Work out the finished part from the listing and answer in its coordinate system (mm). A direction names the side the tool comes from. Round coordinates to 2 decimals unless told otherwise and drop trailing zeros. Write each loop counter-clockwise with the first axis right and the second up, starting at its lowest first coordinate (ties: lowest second). Pieces come first, ordered by that corner, then holes. Notation, with made-up numbers: (-36, 31.5) - (-10, 31.5) arc R6 ccw to (-10, 36.5) - close; hole circle Ø11 at (25.5, 48.5). An arc over 180 degrees is marked (long way). Answer as a JSON object with one key per item and string values.
```python
from build123d import *

# Parameters (mm, degrees)
ESBO_O1_W                  = 69
ESBO_O1_H                  = 31.5
RESSALTO_EXTRUS_O1_DEPTH   = 6
ESBO_O2_W                  = 5
ESBO_O2_H                  = 19
RESSALTO_EXTRUS_O2_DEPTH   = 20
ESBO_O3_W                  = 5
ESBO_O3_H                  = 7
CORTE_EXTRUS_O1_DEPTH      = 10
ESBO_O4_W                  = 4
ESBO_O4_H                  = 31.5
RESSALTO_EXTRUS_O3_DEPTH   = 20
CORTE_EXTRUS_O2_DEPTH      = 4
ESBO_O6_W                  = 4
ESBO_O6_H                  = 6
RESSALTO_EXTRUS_O4_DEPTH   = 50
ESBO_O7_W                  = 4
ESBO_O7_H                  = 63
RESSALTO_EXTRUS_O5_DEPTH   = 10
CORTE_EXTRUS_O3_DEPTH      = 144.957450913
CORTE_EXTRUS_O3_DEPTH_BACK = 144.957450913
ESBO_O8_R                  = 3
ESBO_O13_W                 = 100
ESBO_O13_H                 = 4
RESSALTO_EXTRUS_O6_DEPTH   = 53


with BuildPart() as part:
    # Esboço1 → Ressalto-extrusão1 (new body)
    with BuildSketch(Plane.XY):
        with Locations((-34.5, -15.931977108)):
            Rectangle(ESBO_O1_W, ESBO_O1_H)
    extrude(amount=RESSALTO_EXTRUS_O1_DEPTH)

    # Esboço2 → Ressalto-extrusão2 (add)
    with BuildSketch(Plane.XY.offset(6)):
        with Locations((-60, -22.181977108)):
            Rectangle(ESBO_O2_W, ESBO_O2_H)
    extrude(amount=RESSALTO_EXTRUS_O2_DEPTH)

    # Esboço3 → Corte-extrusão1 (cut)
    with BuildSketch(Plane.XY.offset(26)):
        with Locations((-60, -22.181977108)):
            Rectangle(ESBO_O3_W, ESBO_O3_H)
    extrude(amount=-CORTE_EXTRUS_O1_DEPTH, mode=Mode.SUBTRACT)

    # Esboço4 → Ressalto-extrusão3 (add)
    with BuildSketch(Plane.XY.offset(6)):
        with Locations((-52, -15.931977108)):
            Rectangle(ESBO_O4_W, ESBO_O4_H)
    extrude(amount=RESSALTO_EXTRUS_O3_DEPTH)

    # Esboço5 → Corte-extrusão2 (cut)
    with BuildSketch(Plane(origin=(-50, 0, 0), x_dir=(0, 0, -1), z_dir=(1, 0, 0))):
        Polygon((-22, -25.681977108), (-6, -25.681977108), (-6, -0.181977108), (-22, -0.181977108), (-22, -6.181977108), align=None)
    extrude(amount=-CORTE_EXTRUS_O2_DEPTH, mode=Mode.SUBTRACT)

    # Esboço6 → Ressalto-extrusão4 (add)
    with BuildSketch(Plane(origin=(-50, 0, 0), x_dir=(0, 0, -1), z_dir=(1, 0, 0))):
        with Locations((-24, -28.681977108)):
            Rectangle(ESBO_O6_W, ESBO_O6_H)
    extrude(amount=RESSALTO_EXTRUS_O4_DEPTH)

    # Espelhar10: part across plane


with BuildPart() as part_1:
    add(part.part)
    add(part.part.mirror(Plane.ZX.offset(-0.181977108)))

    # Espelhar11: part across plane


with BuildPart() as part_2:
    add(part_1.part)
    add(part_1.part.mirror(Plane(origin=(0, 0, 0), x_dir=(0, 0, 1), z_dir=(1, 0, 0))))

    # Esboço7 → Ressalto-extrusão5 (add)
    with BuildSketch(Plane(origin=(0, 0, 0), x_dir=(-1, 0, 0), z_dir=(0, 0, -1))):
        with Locations((-67, -0.181977108)):
            Rectangle(ESBO_O7_W, ESBO_O7_H)
    extrude(amount=RESSALTO_EXTRUS_O5_DEPTH)

    # Esboço8 → Corte-extrusão3 (cut, two sides: drawn at the far end of the back side and taken through both)
    with BuildSketch(Plane(origin=(69, 0, 0), x_dir=(0, 0, -1), z_dir=(1, 0, 0)).offset(-CORTE_EXTRUS_O3_DEPTH_BACK)):
        with Locations((5, -0.181977108)):
            Circle(ESBO_O8_R)
    extrude(amount=CORTE_EXTRUS_O3_DEPTH + CORTE_EXTRUS_O3_DEPTH_BACK, mode=Mode.SUBTRACT)

    # Esboço13 → Ressalto-extrusão6 (add)
    with BuildSketch(Plane(origin=(0, -25.681977108, 0), x_dir=(1, 0, 0), z_dir=(0, 1, 0))):
        with Locations((0, -24)):
            Rectangle(ESBO_O13_W, ESBO_O13_H)
    extrude(amount=RESSALTO_EXTRUS_O6_DEPTH)


solid = part_2.part
```
Item 1: A cutting plane is placed at B-B (y = 6). Write down the section's boundary in (x, z), and give its area (3 significant figures).
Results found:
{"outline": "(-69, 0) - (65, 0) - (65, -10) - (69, -10) - (69, 6) - (-69, 6) - close; (-54, 22) - (54, 22) - (54, 26) - (-54, 26) - close", "area": "1,300 mm²"}
Item 2: A cutting plane is placed at A-A (z = -5). Write down the section's boundary in (x, y), and give its area (3 significant figures).
Results found:
{"outline": "(65, -31.68) - (69, -31.68) - (69, -3.18) - (65, -3.18) - close; (65, 2.82) - (69, 2.82) - (69, 31.32) - (65, 31.32) - close", "area": "228 mm²"}
Item 3: Determine the mould class of faces 6 (the flat face through (-60, 28, 26)), 7 (the flat face through (-60, 12.318, 16)), 8 (the flat face through (1, -31.682, 4)) for opening direction Y: pulls with the +Y half, pulls with the -Y half, needs draft (parallel to the pull), parting line crosses it, or undercut.
Results found:
{"face 6": "needs draft", "face 7": "undercut", "face 8": "pulls with the -Y half"}
Item 4: Each of these flat-tipped pins is pushed along its axis until it touches: P1, Ø9.5, axis at y = 26, z = 13.5, coming from the -X side; P2, Ø10, axis at x = -49.5, y = -20, coming from the -Z side; P3, Ø3, axis at x = 44, z = 8.5, coming from the +Y side; P4, Ø6.5, axis at y = 29.5, z = 11.5, coming from the +X side. Where does it stop, or does it pass through?
Results found:
{"P1": "x = -62.5", "P2": "z = 0", "P3": "through", "P4": "x = 62.5"}
Item 5: A cutting plane is placed at D-D (z = 11). Give the number of separate pieces and of enclosed holes in the cut face, and give its area (3 significant figures).
Results found:
{"separate pieces": "8", "enclosed holes": "0", "area": "476 mm²"}
Item 6: A cutting plane is placed at C-C (x = 7.5). Write down the section's boundary in (y, z), and give its area (3 significant figures).
Results found:
{"outline": "(-31.68, 0) - (31.32, 0) - (31.32, 6) - (-31.68, 6) - close; (-31.68, 22) - (31.32, 22) - (31.32, 26) - (-31.68, 26) - close", "area": "630 mm²"}
Item 7: Consider line 1 along X through (y, z) = (-14, 22.5); line 2 along X through (y, z) = (-28, 20.5); line 3 along Z through (x, y) = (-23.5, 7.5). Determine where each line is inside the solid, lowest interval first.
Results found:
{"line 1": "-62.5 to -57.5, -54 to 54, 57.5 to 62.5", "line 2": "-62.5 to -57.5, -54 to -50, 50 to 54, 57.5 to 62.5", "line 3": "0 to 6, 22 to 26"}
Item 8: For faces 1 (the flat face through (52, -25.682, 14)), 2 (the flat face through (-60, -12.682, 16)), 3 (the flat face through (50, -29, 14)), 4 (the flat face through (62.5, -22, 14)), 5 (the flat face through (60, -12.682, 16)), determine the directions among +Z, -Z, +X, -X, +Y, -Y from which every point of the face is accessible in a straight line to the end or side of a thin tool.
Results found:
{"face 1": "none", "face 2": "+Z, -X", "face 3": "+Y, -Y", "face 4": "+Z, +X, +Y, -Y", "face 5": "+Z, +X"}
